Input: part model. Units: mm. Frame: model coordinates. Face numbers are marked on the shaded views. A direction names the side the tool comes from. Give positions to 0.01 mm unless a question says otherwise; leave off trailing zeros. Loops run counter-clockwise (first coordinate to the right, second up) from the corner with the lowest first, then second, coordinate; pieces in that order, holes last. Notation, with made-up numbers: M -29,-25 L 5,-25 A24 ccw 5,-8 Z; hole C 25.25,65 d8. An arc over 180 degrees is marked long. Answer as a JSON object with one key per item and string values. Group by question number.
```python
from build123d import *

# Parameters (mm, degrees)
F1_DEPTH = 17.99844
F3_DEPTH = 17.99944


with BuildPart() as f1:
    # F0 (on Front) → F1 (new body)
    with BuildSketch(Plane.XZ):
        with BuildLine():
            Line((-15.24, 29.099356), (-63.5, 29.099356))
            ThreePointArc((-63.5, 29.099356), (0, -69.85), (63.5, 29.099356))
            Line((63.5, 29.099356), (15.24, 29.099356))
            Line((15.24, 29.099356), (15.24, 47.024507))
            Line((15.24, 47.024507), (-15.24, 47.024507))
            Line((-15.24, 47.024507), (-15.24, 29.099356))
        make_face()
    extrude(amount=F1_DEPTH)

    # F2 (on face) → F3 (cut, through all)
    with BuildSketch(Plane.XZ.offset(17.99844)):
        with BuildLine():
            Line((-7.493, 19.099376), (-56.720708, 19.099376))
            ThreePointArc((-56.720708, 19.099376), (0, -59.85002), (56.720708, 19.099376))
            Line((56.720708, 19.099376), (7.493, 19.099376))
            Line((7.493, 19.099376), (7.493, 47.024507))
            Line((7.493, 47.024507), (-7.493, 47.024507))
            Line((-7.493, 47.024507), (-7.493, 19.099376))
        make_face()
    extrude(amount=-F3_DEPTH, mode=Mode.SUBTRACT)


solid = f1.part
```
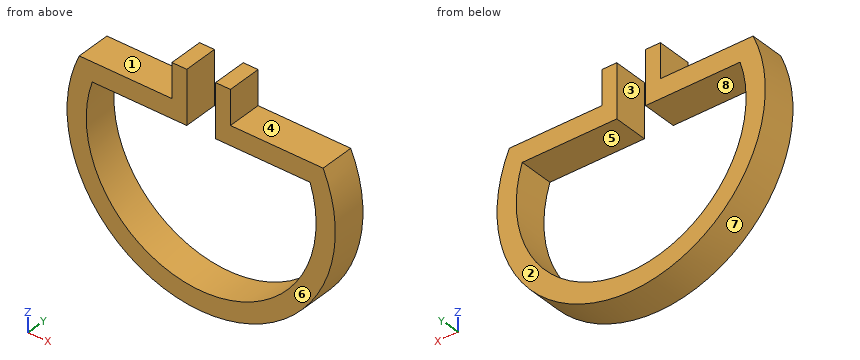
1. Mould query, pull axis Z, two halves, no side actions, for the marked faces 6, 7 and 8. Classes: pulls with the +Z half, pulls with the -Z half, needs draft (parallel to the pull), parting line crosses it, or undercut.
2. First-contact query: P1, Ø5.5, axis at x = 39.5, y = -6.5, coming from the -Z side; P2, Ø5, axis at y = -15, z = -37, coming from the -X side; P3, Ø9, axis at x = -42.5, y = -11, coming from the +Z side. Flat tips, straight axial feed; report the tip coordinate or a pass-through.
3. Section C-C (y = -7.25). Output: boundary loops of the cut face in (x, z).
4. Section D-D (x = 0). Output: boundary loops of the cut face in (y, z).
5. Section A-A (z = 0). Output: boundary loops of the cut face in (x, y).
6. Section B-B (x = 34.5). Output: boundary loops of the cut face in (y, z), then the cut area to 3 significant figures.
7. Material intervals for L1, parallel to X at y = -9, z = 35.5; L2, parallel to X at y = -11.75, z = 0; L3, parallel to Z at x = 0, y = -12.5, sorted ascending.
8. Reachability of the marked faces 1, 2, 3, 4 and 5 from +Z, -Z, +X, -X, +Y, -Y: full face, straight path, thin tool, end or side. Return the list, or none.
Geometry results:
{
 "1": {"face 6": "needs draft", "face 7": "parting line crosses it", "face 8": "undercut"},
 "2": {"P1": "z = -59.4", "P2": "x = -60.74", "P3": "z = 29.1"},
 "3": {"outline": "M -63.5,29.1 A69.85 ccw long 63.5,29.1 L 15.24,29.1 L 15.24,47.02 L 7.49,47.02 L 7.49,19.1 L 56.72,19.1 A59.85 cw long -56.72,19.1 L -7.49,19.1 L -7.49,47.02 L -15.24,47.02 L -15.24,29.1 Z"},
 "4": {"outline": "M -18,-69.85 L 0,-69.85 L 0,-59.85 L -18,-59.85 Z"},
 "5": {"outline": "M -69.85,-18 L -59.85,-18 L -59.85,0 L -69.85,0 Z; M 59.85,-18 L 69.85,-18 L 69.85,0 L 59.85,0 Z"},
 "6": {"outline": "M -18,-60.74 L 0,-60.74 L 0,-48.91 L -18,-48.91 Z; M -18,19.1 L 0,19.1 L 0,29.1 L -18,29.1 Z", "area": "393 mm2"},
 "7": {"L1": "-15.24 to -7.49, 7.49 to 15.24", "L2": "-69.85 to -59.85, 59.85 to 69.85", "L3": "-69.85 to -59.85"},
 "8": {"face 1": "+Z, -X, +Y, -Y", "face 2": "+Z, -Z, +X, -X, +Y", "face 3": "+Z, +Y, -Y", "face 4": "+Z, +X, +Y, -Y", "face 5": "+Y, -Y"}
}
